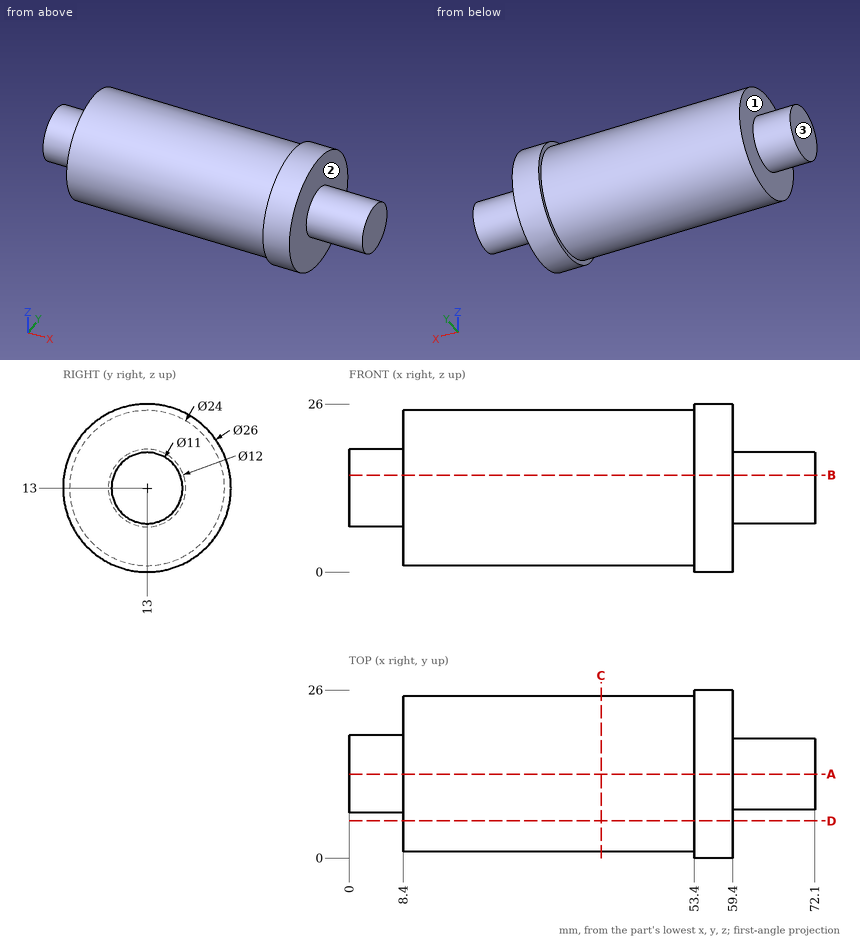
Answer from the drawing. Dimensions are ordinates in mm from the lowest x, y and z of the part. A direction names the side the tool comes from. Round coordinates to 2 decimals unless told otherwise and drop trailing zeros. Write each loop counter-clockwise with the first axis right and the second up, starting at its lowest first coordinate (ties: lowest second). Pieces come first, ordered by that corner, then holes. Notation, with made-up numbers: (-33.5, 61.25) - (-23.5, 61.25) arc R7 cw to (-23.5, 69.25) - close; hole circle Ø5 at (41, 4.5). An arc over 180 degrees is marked (long way). One line per item, written item: value.
Q1. Find section D-D (y = 5.75). Determine the outline of the cut face in (x, z).
The answers:
outline: (8.4, 3.44) - (53.4, 3.44) - (53.4, 2.21) - (59.4, 2.21) - (59.4, 23.79) - (53.4, 23.79) - (53.4, 22.56) - (8.4, 22.56) - close
Q2. Find section C-C (x = 39). Determine the outline of the cut face in (y, z), and give its area (3 significant figures).
The answers:
outline: circle Ø24 at (13, 13)
area: 452 mm2
Q3. Find section B-B (z = 15). Determine the outline of the cut face in (x, y).
The answers:
outline: (0, 7.34) - (8.4, 7.34) - (8.4, 1.17) - (53.4, 1.17) - (53.4, 0.15) - (59.4, 0.15) - (59.4, 7.88) - (72.1, 7.88) - (72.1, 18.12) - (59.4, 18.12) - (59.4, 25.85) - (53.4, 25.85) - (53.4, 24.83) - (8.4, 24.83) - (8.4, 18.66) - (0, 18.66) - close
Q4. Straight lines are drawn through the part: line 1 (X direction, y = 8.5, z = 22); line 2 (X direction, y = 17, z = 17); line 3 (Z direction, x = 56, y = 12). For each, find the intervals that lie inside material, in ascending order. Write a range as from..to.
The answers:
line 1: x = 8.4..59.4
line 2: x = 0..59.4
line 3: z = 0.04..25.96
Q5. Each of these flat-tipped pins is pushed along its axis until it touches: P1, Ø2, axis at y = 22.5, z = 14, coming from the +X side; P2, Ø4, axis at x = 46, y = 9.5, coming from the +Z side; P3, Ø2, axis at x = 63, z = 21, coming from the +Y side; P4, Ø5, axis at x = 43.5, z = 19, coming from the -Y side. Where does it stop, or does it pass through?
The answers:
P1: stops at x = 59.4
P2: stops at z = 24.91
P3: passes through
P4: stops at y = 1.52
Q6. Find section A-A (y = 13). Determine the outline of the cut face in (x, z), and give its area (3 significant figures).
The answers:
outline: (0, 7) - (8.4, 7) - (8.4, 1) - (53.4, 1) - (53.4, 0) - (59.4, 0) - (59.4, 7.5) - (72.1, 7.5) - (72.1, 18.5) - (59.4, 18.5) - (59.4, 26) - (53.4, 26) - (53.4, 25) - (8.4, 25) - (8.4, 19) - (0, 19) - close
area: 1,480 mm2
Q7. Which of the six approach directions +Z, -Z, +X, -X, +Y, -Y give full straight-line access (tool end or side, diameter ignored) to the marked faces 1, 2 and 3?
The answers:
face 1: -X
face 2: +X
face 3: +Z, -Z, -X, +Y, -Y
